```python
from build123d import *

# Parameters (mm, degrees)
F2_DEPTH   = 25.4
F3_SIZE2   = 4.022955
F3_SIZE    = 25.39999
F3_2_SIZE2 = 4.022955
F3_2_SIZE  = 25.39999


# Not quite as in the source:
# - a fillet or chamfer is up to 0.001 mm smaller than in the source, because OpenCascade refuses the exact size


with BuildPart() as f2:
    # F1 (on Top) → F2 (new body)
    with BuildSketch(Plane.XY):
        Polygon((-274.9808599955, 457.2), (-177.8, 0), (177.8, 0), (274.9808599955, 457.2), align=None)
    extrude(amount=F2_DEPTH)

    # F3 (size 25.4 and 4.0229647842 in the source; OpenCascade refuses exactly that, so slightly less here)
    f3_edges = [f2.edges().sort_by_distance(p)[0] for p in [
        (-226.39043, 228.6, 25.4),
    ]]
    f3_side = f2.faces().sort_by_distance((-226.39043, 228.6, 12.7))[0]
    chamfer(f3_edges, length=F3_SIZE, length2=F3_SIZE2, reference=f3_side)

    # F3#2 (size 25.4 and 4.0229647842 in the source; OpenCascade refuses exactly that, so slightly less here)
    f3_2_edges = [f2.edges().sort_by_distance(p)[0] for p in [
        (226.39043, 228.6, 25.4),
    ]]
    f3_2_side = f2.faces().sort_by_distance((226.39043, 228.6, 12.7))[0]
    chamfer(f3_2_edges, length=F3_2_SIZE, length2=F3_2_SIZE2, reference=f3_2_side)


solid = f2.part
```
The model under review builds one solid part; all positions refer to its coordinate system, in mm. Coordinates: 2 decimals unless noted, no trailing zeros. Write each loop counter-clockwise with the first axis right and the second up, starting at its lowest first coordinate (ties: lowest second). Pieces come first, ordered by that corner, then holes.
1) To check wall thickness, follow probe 1 along X at (y, z) = (406.5, 24.25); probe 2 along X at (y, z) = (150, 19.75). State the ranges of each line that lie inside material, in increasing order.
2) We need section C-C on z = 21.5. State the section outline as (x, y) points, then the cut area to 3 significant figures.
3) Clearance check with flat-ended pins moving along their axes: pin 1 Ø12 at (y, z) = (224, 7.5) entering from -X; pin 2 Ø3 at (y, z) = (371, 21.5) entering from +X; pin 3 Ø12 at (y, z) = (382, 11) entering from +X. State where each tip first meets the part, or that it passes through.
Answer list:
1. probe 1: x = -260.28 to 260.28
1. probe 2: x = -206.49 to 206.49
2. outline: (-271.5, 457.2) - (-174.32, 0) - (174.32, 0) - (271.5, 457.2) - close
2. area: 204,000 mm2
3. pin 1: stops at x = -225.8
3. pin 2: stops at x = 253.58
3. pin 3: stops at x = 258.82
